Part model, mm, in its own coordinate system. A direction names the side the tool comes from. Round coordinates to 2 decimals unless told otherwise and drop trailing zeros. Write each loop counter-clockwise with the first axis right and the second up, starting at its lowest first coordinate (ties: lowest second). Pieces come first, ordered by that corner, then holes.
```python
from build123d import *

# Parameters (mm, degrees)
CYLINDER004_R          = 4
CYLINDER004_DEPTH      = 5
ARRAY004_X_COUNT       = 2
ARRAY004_X_PITCH       = 35
CYLINDER003_R          = 3
CYLINDER003_DEPTH      = 10
CYLINDER003_ROLL_ANGLE = 90
ARRAY003_X_COUNT       = 2
ARRAY003_X_PITCH       = 21
CYLINDER001_R          = 1.1
CYLINDER001_DEPTH      = 50
CYLINDER001_ROLL_ANGLE = 90
ARRAY001_X_COUNT       = 2
ARRAY001_X_PITCH       = 21
ARRAY001_Z_COUNT       = 2
ARRAY001_Z_PITCH       = 12.2
CYLINDER002_R          = 1.6
CYLINDER002_DEPTH      = 10
ARRAY002_X_COUNT       = 2
ARRAY002_X_PITCH       = 35
BOX001_W               = 28
BOX001_H               = 2.5
BOX001_DEPTH           = 21
FILLET001_R            = 3
BOX002_W               = 44
BOX002_H               = 12
BOX002_DEPTH           = 2.5
FILLET_R               = 3
FILLET002_R            = 2


with BuildPart() as array004:
    # Cylinder004 → Cylinder004 (new body)
    with BuildSketch(Plane(origin=(-17.5, 0, 2.5), x_dir=(1, 0, 0), z_dir=(0, 0, 1))):
        Circle(CYLINDER004_R)
    extrude(amount=CYLINDER004_DEPTH)

    # Array004 X: Array004 ×2


with BuildPart() as array004_1:
    add(array004.part)
    with Locations(*[(i * ARRAY004_X_PITCH, 0, 0) for i in range(1, ARRAY004_X_COUNT)]):
        add(array004.part)


with BuildPart() as array003:
    # Cylinder003 → Cylinder003 (new body)
    with BuildSketch(Plane.XY):
        Circle(CYLINDER003_R)
    extrude(amount=CYLINDER003_DEPTH)


with BuildPart() as array003_1:
    # Cylinder003 roll: moved
    add(array003.part.rotate(Axis((0, 0, 0), (1, 0, 0)), CYLINDER003_ROLL_ANGLE))


with BuildPart() as array003_2:
    # Cylinder003 placement: moved
    add(array003_1.part.moved(Location((-10.5, 6.5, 6))))

    # Array003 X: Array003 ×2


with BuildPart() as array003_3:
    add(array003_2.part)
    with Locations(*[(i * ARRAY003_X_PITCH, 0, 0) for i in range(1, ARRAY003_X_COUNT)]):
        add(array003_2.part)


with BuildPart() as array001:
    # Cylinder001 → Cylinder001 (new body)
    with BuildSketch(Plane.XY):
        Circle(CYLINDER001_R)
    extrude(amount=CYLINDER001_DEPTH)


with BuildPart() as array001_1:
    # Cylinder001 roll: moved
    add(array001.part.rotate(Axis((0, 0, 0), (1, 0, 0)), CYLINDER001_ROLL_ANGLE))


with BuildPart() as array001_2:
    # Cylinder001 placement: moved
    add(array001_1.part.moved(Location((-10.5, 20, 6))))

    # Array001 X: Array001 ×2


with BuildPart() as array001_3:
    add(array001_2.part)
    with Locations(*[(i * ARRAY001_X_PITCH, 0, 0) for i in range(1, ARRAY001_X_COUNT)]):
        add(array001_2.part)

    # Array001 Z: Array001 ×2


with BuildPart() as array001_4:
    add(array001_3.part)
    with Locations(*[(0, 0, i * ARRAY001_Z_PITCH) for i in range(1, ARRAY001_Z_COUNT)]):
        add(array001_3.part)


with BuildPart() as fusion001:
    # Cylinder002 → Cylinder002 (new body)
    with BuildSketch(Plane(origin=(-17.5, 0, -1), x_dir=(1, 0, 0), z_dir=(0, 0, 1))):
        Circle(CYLINDER002_R)
    extrude(amount=CYLINDER002_DEPTH)

    # Array002 X: Fusion001 ×2


with BuildPart() as fusion001_1:
    add(fusion001.part)
    with Locations(*[(i * ARRAY002_X_PITCH, 0, 0) for i in range(1, ARRAY002_X_COUNT)]):
        add(fusion001.part)

    # Fusion001: union Array001
    add(array001_4.part)


with BuildPart() as fillet001:
    # Box001 → Box001 (new body)
    with BuildSketch(Plane(origin=(-14, -6, 0), x_dir=(1, 0, 0), z_dir=(0, 0, 1))):
        with Locations((14, 1.25)):
            Rectangle(BOX001_W, BOX001_H)
    extrude(amount=BOX001_DEPTH)

    # Fillet001
    fillet001_edges = [fillet001.edges().sort_by_distance(p)[0] for p in [
        (-14, -4.75, 21),
        (14, -4.75, 21),
    ]]
    fillet(fillet001_edges, radius=FILLET001_R)


with BuildPart() as cut002006002006:
    # Box002 → Box002 (new body)
    with BuildSketch(Plane(origin=(-22, -6, 0), x_dir=(1, 0, 0), z_dir=(0, 0, 1))):
        with Locations((22, 6)):
            Rectangle(BOX002_W, BOX002_H)
    extrude(amount=BOX002_DEPTH)

    # Fillet
    fillet_edges = [cut002006002006.edges().sort_by_distance(p)[0] for p in [
        (-22, -6, 1.25),
        (-22, 6, 1.25),
        (22, -6, 1.25),
        (22, 6, 1.25),
    ]]
    fillet(fillet_edges, radius=FILLET_R)

    # Fusion: union Fillet001
    add(fillet001.part)

    # Fillet002
    fillet002_edges = [cut002006002006.edges().sort_by_distance(p)[0] for p in [
        (14, -4.75, 2.5),
        (0, -3.5, 2.5),
        (-14, -4.75, 2.5),
    ]]
    fillet(fillet002_edges, radius=FILLET002_R)

    # Cut002006002004: cut Fusion001
    add(fusion001_1.part, mode=Mode.SUBTRACT)

    # Cut002006002005: cut Array003
    add(array003_3.part, mode=Mode.SUBTRACT)

    # Cut002006002006: cut Array004
    add(array004_1.part, mode=Mode.SUBTRACT)


solid = cut002006002006.part
```
Q1. Drop flat-ended pins along their axis: pin 1 (6 mm diameter, centred on y = 1.5, z = 17, fed in from +X); pin 2 (0.8 mm diameter, centred on y = -4.5, z = 12, fed in from +X); pin 3 (6 mm diameter, centred on x = 2, y = 2.5, fed in from +Z); pin 4 (1.5 mm diameter, centred on y = -3.5, z = 4.5, fed in from -X). Give the stop position or say it passes through.
Values follow:
pin 1: passes through
pin 2: stops at x = 14
pin 3: stops at z = 2.5
pin 4: stops at x = -14.15
Q2. Mould opens along X. For faces 4 (the cylindrical face through (16.32, 1.08, 1.23)), 5 (the flat face through (22, 0, 1)), 6 (the cylindrical face through (-14.677, -2.834, 2.695)) say: +X half, -X half, draft (parallel to the pull), parting line (faces both ways), or undercut.
Values follow:
face 4: undercut
face 5: +X half
face 6: -X half
Q3. Cut at B-B on x = -17.5. Write the cut outline in (y, z), plus the area to 3 significant figures.
Values follow:
outline: (-6, 0) - (-1.6, 0) - (-1.6, 2.5) - (-6, 2.5) - close; (1.6, 0) - (6, 0) - (6, 2.5) - (1.6, 2.5) - close
area: 22.0 mm2
Q4. Cut at D-D on z = 6.5. Write the cut outline in (x, y).
Values follow:
outline: (-14, -6) - (-11.48, -6) - (-11.48, -3.5) - (-14, -3.5) - close; (-9.52, -6) - (9.52, -6) - (9.52, -3.5) - (-9.52, -3.5) - close; (11.48, -6) - (14, -6) - (14, -3.5) - (11.48, -3.5) - close
Q5. Cut at C-C on y = 0. Write the cut outline in (x, z), plus the area to 3 significant figures.
Values follow:
outline: (-22, 0) - (-19.1, 0) - (-19.1, 2.5) - (-22, 2.5) - close; (-15.9, 0) - (15.9, 0) - (15.9, 2.5) - (-15.9, 2.5) - close; (19.1, 0) - (22, 0) - (22, 2.5) - (19.1, 2.5) - close
area: 94.0 mm2
Q6. Cut at A-A on x = -10.5. Write the cut outline in (y, z), plus the area to 3 significant figures.
Values follow:
outline: (-6, 0) - (6, 0) - (6, 2.5) - (-1.5, 2.5) arc R2 cw to (-2.82, 3) - (-3.5, 3) - (-3.5, 4.9) - (-6, 4.9) - close; (-6, 7.1) - (-3.5, 7.1) - (-3.5, 17.1) - (-6, 17.1) - close; (-6, 19.3) - (-3.5, 19.3) - (-3.5, 21) - (-6, 21) - close
area: 65.8 mm2
Q7. Which spindle directions (+Z, -Z, +X, -X, +Y, -Y) get a long thin tool onto all of the face, cutting with end or side? Do faces 1 (the flat face through (14, -5, 11)), 2 (the flat face through (-14, -5, 11)), 3 (the cylindrical face through (-10.5, -3.2, 3)). Say none if no direction does.
Values follow:
face 1: +Z, +X, +Y, -Y
face 2: +Z, -X, +Y, -Y
face 3: +Z, +Y
Q8. Wall check: L1, parallel to Z at x = 10.5, y = -4.1; L2, parallel to X at y = 0, z = 1.95; L3, parallel to X at y = -0.5, z = 1. Give the ranges that are in metal, low to high.
Values follow:
L1: z = 0 to 4.9, 7.1 to 17.1, 19.3 to 21
L2: x = -22 to -19.1, -15.9 to 15.9, 19.1 to 22
L3: x = -22 to -19.02, -15.98 to 15.98, 19.02 to 22
